Part model, mm, in its own coordinate system. Coordinates: 2 decimals unless noted, no trailing zeros. Order: outer loops, then holes, each group sorted by start corner. A loop starts at its lowest first (then second) coordinate and runs counter-clockwise, first axis right, second up.
```python
from build123d import *

# Parameters (mm, degrees)
SKETCH_1_R      = 1.225
EXTRUDE_1_DEPTH = 10
SKETCH_1_7_R    = 1.25
EXTRUDE_2_DEPTH = 2.5
FILLET_1_R      = 3


with BuildPart() as part:
    # Sketch 1 → Extrude 1 (new body)
    with BuildSketch(Plane(origin=(0, 0, 0), x_dir=(1, 0, 0), z_dir=(0, 1, 0))):
        with BuildLine():
            Line((22.5, 10.1), (-22.5, 10.1))
            ThreePointArc((-22.5, 10.1), (-26.035533906, 8.635533906), (-27.5, 5.1))
            Line((-27.5, 5.1), (-27.5, -5.1))
            ThreePointArc((-27.5, -5.1), (-26.035533906, -8.635533906), (-22.5, -10.1))
            Line((-22.5, -10.1), (22.5, -10.1))
            ThreePointArc((22.5, -10.1), (26.035533906, -8.635533906), (27.5, -5.1))
            Line((27.5, -5.1), (27.5, 5.1))
            ThreePointArc((27.5, 5.1), (26.035533906, 8.635533906), (22.5, 10.1))
        make_face()
        with Locations(Location((-22, 0, 0), (0, 0, 270))):
            Circle(SKETCH_1_R, mode=Mode.SUBTRACT)
        with Locations(Location((22, 0, 0), (0, 0, 270))):
            Circle(SKETCH_1_R, mode=Mode.SUBTRACT)
        with Locations(Location((-16, 0, 0), (0, 0, 270))):
            Circle(SKETCH_1_R, mode=Mode.SUBTRACT)
        with Locations(Location((16, 0, 0), (0, 0, 270))):
            Circle(SKETCH_1_R, mode=Mode.SUBTRACT)
        with BuildLine():
            ThreePointArc((-3.2, 0.894427191), (-4, 0), (-3.2, -0.894427191))
            Line((-3.2, -0.894427191), (-3.2, -3.2))
            Line((-3.2, -3.2), (3.2, -3.2))
            Line((3.2, -3.2), (3.2, -0.894427191))
            ThreePointArc((3.2, -0.894427191), (4, 0), (3.2, 0.894427191))
            Line((3.2, 0.894427191), (3.2, 2.141421356))
            Line((3.2, 2.141421356), (2.141421356, 3.2))
            Line((2.141421356, 3.2), (-2.141421356, 3.2))
            Line((-2.141421356, 3.2), (-3.2, 2.141421356))
            Line((-3.2, 2.141421356), (-3.2, 0.894427191))
        make_face(mode=Mode.SUBTRACT)
    extrude(amount=EXTRUDE_1_DEPTH)

    # Sketch 1_7 → Extrude 2 (add)
    with BuildSketch(Plane(origin=(0, 0, 0), x_dir=(1, 0, 0), z_dir=(0, 1, 0))):
        with BuildLine():
            Line((-3.2, 0.894427191), (-3.2, 2.141421356))
            Line((-3.2, 2.141421356), (-2.141421356, 3.2))
            Line((-2.141421356, 3.2), (2.141421356, 3.2))
            Line((2.141421356, 3.2), (3.2, 2.141421356))
            Line((3.2, 2.141421356), (3.2, 0.894427191))
            ThreePointArc((3.2, 0.894427191), (4, 0), (3.2, -0.894427191))
            Line((3.2, -0.894427191), (3.2, -3.2))
            Line((3.2, -3.2), (-3.2, -3.2))
            Line((-3.2, -3.2), (-3.2, -0.894427191))
            ThreePointArc((-3.2, -0.894427191), (-4, 0), (-3.2, 0.894427191))
        make_face()
        with Locations(Location((0, 0, 0), (0, 0, 270))):
            Circle(SKETCH_1_7_R, mode=Mode.SUBTRACT)
    extrude(amount=EXTRUDE_2_DEPTH)

    # Fillet 1
    fillet_1_edges = [part.edges().sort_by_distance(p)[0] for p in [
        (0, 10, 10.1),
        (26.035533906, 10, 8.635533906),
        (27.5, 10, 0),
        (26.035533906, 10, -8.635533906),
        (0, 10, -10.1),
        (-26.035533906, 10, -8.635533906),
        (-27.5, 10, 0),
        (-26.035533906, 10, 8.635533906),
    ]]
    fillet(fillet_1_edges, radius=FILLET_1_R)


solid = part.part
```
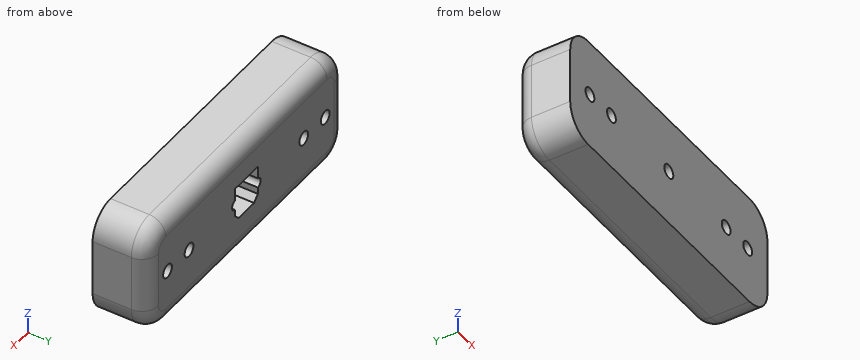
(1) Slice it at C-C, the plane z = 2.25. Give the cut face in (x, y), then the cut area to 3 significant figures.
(2) Slice it at B-B, the plane x = 16. Give the cut face in (y, z) (3 decimals), then the cut area to 3 significant figures.
(3) Drop flat-ended pins along their axis: pin 1 (1.5 mm diameter, centred on x = 22, z = 0, fed in from +Y); pin 2 (1.9 mm diameter, centred on x = 0, z = 1, fed in from +Y); pin 3 (1.8 mm diameter, centred on y = 7.5, z = 1.5, fed in from -X). Give the stop position or say it passes through.
(4) Slice it at D-D, the plane y = 1.5. Give the cut face in (x, z) (3 decimals), then the cut area to 3 significant figures.
(5) Probe line 1 (X direction, y = 2.25, z = 0) (3 decimals); line 2 (X direction, y = 7.25, z = 0) (3 decimals); line 3 (Y direction, x = 3, z = 0.25). List the from-to ranges inside material, lowest first.
(6) Slice it at A-A, the plane y = 4.25. Give the cut face in (x, z) (3 decimals), then the cut area to 3 significant figures.
Here are the results:
1. outline: (-27.5, 0) - (27.5, 0) - (27.5, 7) arc R3 ccw to (24.5, 10) - (3.2, 10) - (3.2, 2.5) - (-3.2, 2.5) - (-3.2, 10) - (-24.5, 10) arc R3 ccw to (-27.5, 7) - close
1. area: 498 mm2
2. outline: (0, -10.1) - (7, -10.1) arc R3 ccw to (10, -7.1) - (10, -1.225) - (0, -1.225) - close; (0, 1.225) - (10, 1.225) - (10, 7.1) arc R3 ccw to (7, 10.1) - (0, 10.1) - close
2. area: 174 mm2
3. pin 1: passes through
3. pin 2: stops at y = 2.5
3. pin 3: stops at x = -27.5
4. outline: (-27.5, -5.1) arc R5 ccw to (-22.5, -10.1) - (22.5, -10.1) arc R5 ccw to (27.5, -5.1) - (27.5, 5.1) arc R5 ccw to (22.5, 10.1) - (-22.5, 10.1) arc R5 ccw to (-27.5, 5.1) - close; hole circle Ø2.45 at (-22, 0); hole circle Ø2.45 at (-16, 0); hole circle Ø2.5 at (0, 0); hole circle Ø2.45 at (16, 0); hole circle Ø2.45 at (22, 0)
4. area: 1,070 mm2
5. line 1: x = -27.5 to -23.225, -20.775 to -17.225, -14.775 to -1.25, 1.25 to 14.775, 17.225 to 20.775, 23.225 to 27.5
5. line 2: x = -27.49 to -23.225, -20.775 to -17.225, -14.775 to -4, 4 to 14.775, 17.225 to 20.775, 23.225 to 27.49
5. line 3: y = 0 to 2.5
6. outline: (-27.5, -5.1) arc R5 ccw to (-22.5, -10.1) - (22.5, -10.1) arc R5 ccw to (27.5, -5.1) - (27.5, 5.1) arc R5 ccw to (22.5, 10.1) - (-22.5, 10.1) arc R5 ccw to (-27.5, 5.1) - close; hole circle Ø2.45 at (-22, 0); hole circle Ø2.45 at (-16, 0); hole (-3.2, -2.141) - (-2.141, -3.2) - (2.141, -3.2) - (3.2, -2.141) - (3.2, -0.894) arc R0.9 ccw to (3.2, 0.894) - (3.2, 3.2) - (-3.2, 3.2) - (-3.2, 0.894) arc R0.9 ccw to (-3.2, -0.894) - close; hole circle Ø2.45 at (16, 0); hole circle Ø2.45 at (22, 0)
6. area: 1,030 mm2
